from build123d import *

# Parameters (mm, degrees)
CROQUIS1_W                        = 50
CROQUIS1_H                        = 39.9
SALIENTE_EXTRUIR1_DEPTH           = 22.5
VACIADO1_T                        = -4
CORTAR_EXTRUIR1_START             = -9.2
CORTAR_EXTRUIR1_DEPTH             = 3.5
CORTAR_EXTRUIR3_REACH             = 41.9
CROQUIS4_R                        = 1
CORTAR_EXTRUIR3_DIRECTION_2_DEPTH = 1
CROQUIS5_R                        = 1
CORTAR_EXTRUIR4_DEPTH             = 5
CORTAR_EXTRUIR5_DEPTH             = 12
CROQUIS8_W                        = 11.85
CROQUIS8_H                        = 3
CORTAR_EXTRUIR6_DEPTH             = 1
CORTAR_EXTRUIR6_DEPTH_BACK        = 46
REDONDEO1_R                       = 4


with BuildPart() as part:
    # Croquis1 → Saliente-Extruir1 (new body, symmetric)
    with BuildSketch(Plane(origin=(0, 0, 0), x_dir=(0, 0, -1), z_dir=(1, 0, 0))):
        Rectangle(CROQUIS1_W, CROQUIS1_H)
    extrude(amount=SALIENTE_EXTRUIR1_DEPTH, both=True)

    # Vaciado1
    vaciado1_openings = [part.faces().sort_by_distance(p)[0] for p in [
        (0, 0, 25),
    ]]
    offset(amount=VACIADO1_T, openings=vaciado1_openings, kind=Kind.INTERSECTION)

    # Croquis2 → Cortar-Extruir1 (cut)
    with BuildSketch(Plane(origin=(0, 19.95, 0), x_dir=(1, 0, 0), z_dir=(0, 1, 0)).offset(CORTAR_EXTRUIR1_START)):
        Polygon((-22.5, 25), (-5.9, 25), (-5.9, 21), (-18.5, 21), (-18.5, 0), (-22.5, 0), align=None)
        Polygon((18.5, 0), (22.5, 0), (22.5, 25), (5.9, 25), (5.9, 21), (18.5, 21), align=None)
    extrude(amount=CORTAR_EXTRUIR1_DEPTH, mode=Mode.SUBTRACT)

    # Croquis4 → Cortar-Extruir3 (cut, up to next)
    with BuildSketch(Plane(origin=(0, 19.95, 0), x_dir=(1, 0, 0), z_dir=(0, 1, 0)), mode=Mode.PRIVATE) as cortar_extruir3_sk1:
        Circle(CROQUIS4_R)
    cortar_extruir3_tool1 = extrude(cortar_extruir3_sk1.sketch, amount=-CORTAR_EXTRUIR3_REACH, mode=Mode.PRIVATE) & part.part
    add(cortar_extruir3_tool1.solids().sort_by_distance((0, 19.95, 0))[0], mode=Mode.SUBTRACT)

    # Croquis4 → Cortar-Extruir3 direction 2 (cut)
    with BuildSketch(Plane(origin=(0, 19.95, 0), x_dir=(1, 0, 0), z_dir=(0, 1, 0))):
        Circle(CROQUIS4_R)
    extrude(amount=CORTAR_EXTRUIR3_DIRECTION_2_DEPTH, mode=Mode.SUBTRACT)

    # Croquis5 → Cortar-Extruir4 (cut)
    with BuildSketch(Plane.XY.offset(25)):
        with Locations((0, 17.95)):
            Circle(CROQUIS5_R)
    extrude(amount=-CORTAR_EXTRUIR4_DEPTH, mode=Mode.SUBTRACT)

    # Croquis7 → Cortar-Extruir5 (cut)
    with BuildSketch(Plane(origin=(0, 19.95, 0), x_dir=(1, 0, 0), z_dir=(0, 1, 0))):
        Polygon((5.9, 0), (18.5, 0), (22.5, 0), (22.5, 25), (5.9, 25), (3.9, 25), (3.9, 0), align=None)
    extrude(amount=-CORTAR_EXTRUIR5_DEPTH, mode=Mode.SUBTRACT)

    # Croquis8 → Cortar-Extruir6 (cut, two sides)
    with BuildSketch(Plane.ZY.offset(22.5)) as cortar_extruir6_sk:
        with Locations((-14.875, 1.05)):
            Rectangle(CROQUIS8_W, CROQUIS8_H)
    extrude(amount=CORTAR_EXTRUIR6_DEPTH, mode=Mode.SUBTRACT)
    extrude(cortar_extruir6_sk.sketch, amount=-CORTAR_EXTRUIR6_DEPTH_BACK, mode=Mode.SUBTRACT)

    # Redondeo1
    redondeo1_edges = [part.edges().sort_by_distance(p)[0] for p in [
        (-22.5, 17.1, -25),
        (22.5, -6, -25),
        (-22.5, -4.6, -25),
    ]]
    fillet(redondeo1_edges, radius=REDONDEO1_R)


solid = part.part
Could you check a few things on this model? Use its own coordinates, in mm. A direction names the side the tool comes from. Give positions to 0.01 mm unless a question says otherwise; leave off trailing zeros. Order: outer loops, then holes, each group sorted by start corner. A loop starts at its lowest first (then second) coordinate and runs counter-clockwise, first axis right, second up. Notation, with made-up numbers: (39, 68.25) - (67, 68.25) arc R16 ccw to (67, 86.25) - close; hole circle Ø3 at (-28.75, 69.25). An arc over 180 degrees is marked (long way). One line per question, with ' | ' between items. Start each with the question number.
Item 1: I need wall thicknesses on probe 1 along Y at (x, z) = (0, 21.75); probe 2 along X at (y, z) = (-8, 9.5); probe 3 along Y at (x, z) = (-18, 0.5). Which ranges of each line are inside material? Lowest first, please. Write a range as [from, to].
Item 2: I want a section at C-C on y = 9.5. Write out the boundary of the cut face in (x, z), then the cut area to 3 significant figures.
Item 3: I'm going to push flat-ended pins straight in: pin 1 Ø4.5 at (x, z) = (21.5, -14.5) entering from +Y; pin 2 Ø1.8 at (x, z) = (0, 0) entering from +Y; pin 3 Ø0.9 at (x, y) = (-20, 0.5) entering from -Z. Where does each tip first touch, or does it pass through?
Item 4: I want a section at D-D on y = 17.95. Write out the boundary of the cut face in (x, z).
Item 5: I want a section at B-B on z = 6. Write out the boundary of the cut face in (x, y).
Item 6: Thinking about a two-plate mould opening in Z: for faces 4 (the flat face through (-22.5, 0, 2)), 5 (the flat face through (0, 18, 20)), 6 (the flat face through (20, -0.45, -15)), 7 (the flat face through (-20, 12, 0)), which applies, pulls with the +Z half, pulls with the -Z half, needs draft (parallel to the pull), parting line crosses it, or undercut?
Item 7: For faces 1 (the flat face through (-4, 15.95, 7)), 2 (the flat face through (-21, 1, -20.8)), 3 (the flat face through (19, 7.95, -18)), which set-ups out of +Z, -Z, +X, -X, +Y, -Y let a thin tool reach every point of the face, with its end or its side?
Item 8: I want a section at A-A on x = 0. Write out the boundary of the cut face in (y, z).
Verdict:
1) probe 1: [-19.95, -15.95], [15.95, 16.95], [18.95, 19.95] | probe 2: [-22.5, -18.5], [18.5, 22.5] | probe 3: [-19.95, -15.95], [15.95, 19.95]
2) outline: (-22.5, -21) arc R4 ccw to (-18.5, -25) - (3.9, -25) - (3.9, -21) - (-18.5, -21) - (-18.5, 25) - (-22.5, 25) - close; (18.5, 0) - (22.5, 0) - (22.5, 25) - (18.5, 25) - close | area: 386 mm^2
3) pin 1: y = 7.95 | pin 2: y = -15.95 | pin 3: z = -24.86
4) outline: (-22.5, -21) arc R4 ccw to (-18.5, -25) - (3.9, -25) - (3.9, 0) - (22.5, 0) - (22.5, 25) - (1, 25) - (1, 20) - (-1, 20) - (-1, 25) - (-22.5, 25) - close; hole circle Ø2 at (0, 0)
5) outline: (-22.5, -19.95) - (22.5, -19.95) - (22.5, 19.95) - (-22.5, 19.95) - close; hole (-18.5, -15.95) - (18.5, -15.95) - (18.5, 15.95) - (-18.5, 15.95) - close
6) face 4: needs draft | face 5: pulls with the +Z half | face 6: undercut | face 7: pulls with the -Z half
7) face 1: +Z | face 2: +X, -X | face 3: -Z, +X, +Y
8) outline: (-19.95, -25) - (19.95, -25) - (19.95, -1) - (15.95, -1) - (15.95, -21) - (-15.95, -21) - (-15.95, 25) - (-19.95, 25) - close; (15.95, 1) - (19.95, 1) - (19.95, 25) - (18.95, 25) - (18.95, 20) - (16.95, 20) - (16.95, 25) - (15.95, 25) - close
